Work out the finished part from the listing and answer in its coordinate system (mm). Face numbers are marked on the shaded views. Give positions to 0.01 mm unless a question says otherwise; leave off trailing zeros. Order: outer loops, then holes, each group sorted by start corner. A loop starts at its lowest first (then second) coordinate and runs counter-clockwise, first axis right, second up. Notation, with made-up numbers: (44, 39) - (75, 39) arc R34 cw to (75, 70) - close; hole circle Ø8 at (22.5, 81.25). An arc over 180 degrees is marked (long way). Put each result on its own line as item: value.
```python
from build123d import *

# Parameters (mm, degrees)
F0_R     = 1.7
F0_R_2   = 1.5
F1_DEPTH = 54.45
F2_R     = 1.7
F2_R_2   = 6
F3_DEPTH = 44
F4_R     = 1.7
F4_R_2   = 6
F5_DEPTH = 44
F6_R     = 5
F7_DEPTH = 55
F8_DEPTH = 5


with BuildPart() as f1:
    # F0 (on Top) → F1 (new body)
    with BuildSketch(Plane.XY):
        with BuildLine():
            Line((18.5, 22), (-22, 22))
            Line((-22, 22), (-22, -22))
            Line((-22, -22), (22, -22))
            Line((22, -22), (22, 18))
            Line((22, 18), (21.5, 18))
            ThreePointArc((21.5, 18), (16.37868, 15.87868), (18.5, 21))
            Line((18.5, 21), (18.5, 22))
        make_face()
        with Locations((-17, -10)):
            Circle(F0_R, mode=Mode.SUBTRACT)
        with Locations((0, -15.5)):
            Circle(F0_R_2, mode=Mode.SUBTRACT)
        with Locations((3, -10)):
            Circle(F0_R, mode=Mode.SUBTRACT)
        with Locations((-17, -10)):
            Circle(F0_R)
        with Locations((0, -15.5)):
            Circle(F0_R_2)
        with Locations((3, -10)):
            Circle(F0_R)
    extrude(amount=-F1_DEPTH)

    # F2 (on face) → F3 (cut)
    with BuildSketch(Plane.XZ.offset(22)):
        with Locations((-12, -25)):
            Circle(F2_R)
        with Locations((12, -25)):
            Circle(F2_R)
        with Locations((-7, -12)):
            Circle(F2_R_2)
        with Locations((7, -12)):
            Circle(F2_R_2)
    extrude(amount=-F3_DEPTH, mode=Mode.SUBTRACT)

    # F4 (on face) → F5 (cut)
    with BuildSketch(Plane.YZ.offset(22)):
        with Locations((-12, -12)):
            Circle(F4_R)
        with Locations((12, -12)):
            Circle(F4_R)
        with Locations((-7, -25)):
            Circle(F4_R_2)
        with Locations((7, -25)):
            Circle(F4_R_2)
    extrude(amount=-F5_DEPTH, mode=Mode.SUBTRACT)

    # F6
    f6_edges = [f1.edges().sort_by_distance(p)[0] for p in [
        (22, -22, -27.225),
        (-22, -22, -27.225),
        (-22, 22, -27.225),
    ]]
    fillet(f6_edges, radius=F6_R)

    # F0 (on Top) → F7 (cut)
    with BuildSketch(Plane.XY):
        with Locations((0, -15.5)):
            Circle(F0_R_2)
    extrude(amount=-F7_DEPTH, mode=Mode.SUBTRACT)

    # F0 (on Top) → F8 (cut)
    with BuildSketch(Plane.XY):
        with Locations((-17, -10)):
            Circle(F0_R)
        with Locations((3, -10)):
            Circle(F0_R)
    extrude(amount=-F8_DEPTH, mode=Mode.SUBTRACT)


solid = f1.part
```
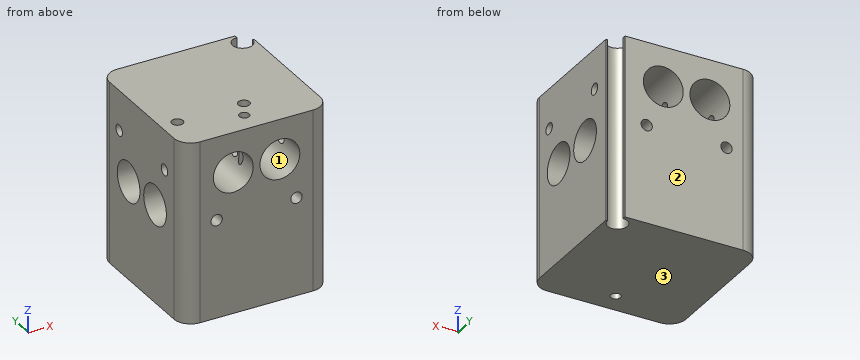
(1) Section C-C, the plane z = -39 is taken. Write down the section's boundary in (x, y), then the cut area to 3 significant figures.
Geometry check:
outline: (-22, -17) arc R5 ccw to (-17, -22) - (17, -22) arc R5 ccw to (22, -17) - (22, 18) - (21.5, 18) arc R3 cw (long way) to (18.5, 21) - (18.5, 22) - (-17, 22) arc R5 ccw to (-22, 17) - close; hole circle Ø3 at (0, -15.5)
area: 1,880 mm²
(2) Determine the mould class of the marked faces 1, 2 and 3 for opening direction Z: pulls with the +Z half, pulls with the -Z half, needs draft (parallel to the pull), parting line crosses it, or undercut.
Geometry check:
face 1: undercut
face 2: needs draft
face 3: pulls with the -Z half
(3) Straight lines are drawn through the part: line 1 (Y direction, x = -15.75, z = -12); line 2 (Y direction, x = -18, z = -22). For each, find the intervals that lie inside material, in ascending order.
Geometry check:
line 1: y = -22 to -13.7, -10.3 to 10.3, 13.7 to 22
line 2: y = -21.9 to -12.2, -1.8 to 1.8, 12.2 to 21.9
(4) Given pin 1 (2 mm diameter, centred on y = -12, z = -12, fed in from -X); pin 2 (0.8 mm diameter, centred on y = 21.5, z = -18.5, fed in from +X), each flat-ended and moving along its own axis, determine where each tip first touches the part or whether it passes through.
Geometry check:
pin 1: passes through
pin 2: stops at x = 18.5
(5) Section D-D, the plane y = -4 is taken. Write down the section's boundary in (x, z), then the cut area to 3 significant figures.
Geometry check:
outline: (-22, -54.45) - (22, -54.45) - (22, -30.2) - (-22, -30.2) - close; (-22, -19.8) - (22, -19.8) - (22, 0) - (-22, 0) - close; hole circle Ø12 at (-7, -12); hole circle Ø12 at (7, -12)
area: 1,710 mm²
(6) Section B-B, the plane x = 0 is taken. Write down the section's boundary in (y, z), then the cut area to 3 significant figures.
Geometry check:
outline: (-22, -54.45) - (-17, -54.45) - (-17, 0) - (-22, 0) - close; (-14, -54.45) - (22, -54.45) - (22, 0) - (-14, 0) - close; hole circle Ø3.4 at (-12, -12); hole circle Ø12 at (-7, -25); hole circle Ø12 at (7, -25); hole circle Ø3.4 at (12, -12)
area: 1,990 mm²
(7) Section A-A, the plane x = 7 is taken. Write down the section's boundary in (y, z), then the cut area to 3 significant figures.
Geometry check:
outline: (-22, -54.45) - (22, -54.45) - (22, -18) - (-22, -18) - close; (-22, -6) - (22, -6) - (22, 0) - (-22, 0) - close; hole circle Ø12 at (-7, -25); hole circle Ø12 at (7, -25)
area: 1,640 mm²
